Verification items for the finished model (mm, model axes). Give positions to 0.01 mm unless a question says otherwise; leave off trailing zeros. Write each loop counter-clockwise with the first axis right and the second up, starting at its lowest first coordinate (ties: lowest second). Pieces come first, ordered by that corner, then holes. Notation, with made-up numbers: (78.25, -37) - (105.25, -37) arc R15 cw to (105.25, -19) - close; hole circle Ø4 at (-28, 38). An arc over 180 degrees is marked (long way). Put each result on its own line as item: value.
Autodesk Inventor part; units mm, degrees
ref_plane "YZ Plane" through (0, 0, 0) normal (1, 0, 0) x (0, 1, 0)
ref_plane "XZ Plane" through (0, 0, 0) normal (0, 1, 0) x (-1, 0, 0)
ref_plane "XY Plane" through (0, 0, 0) normal (0, 0, 1) x (1, 0, 0)
sketch "Sketch1" plane through (0, 0, 0) normal (0, 1, 0) x (-1, 0, 0)
  circle A0 centre (0, 0) radius 25
  circle A1 centre (0, 0) radius 3
  circle A2 centre (0, 18.36) radius 1
  circle A3 centre (-12.9825, 12.9825) radius 1
  circle A4 centre (-18.36, 0) radius 1
  circle A5 centre (-12.9825, -12.9825) radius 1
  circle A6 centre (0, -18.36) radius 1
  circle A7 centre (12.9825, -12.9825) radius 1
  circle A8 centre (18.36, 0) radius 1
  circle A9 centre (12.9825, 12.9825) radius 1
  dimension "d0" = 50
  dimension "d1" = 6
  dimension "d2" = 2
  dimension "d3" = 18.36
  dimension "d6" = 360
extrude "Extrusion1" add sketch "Sketch1" along normal blind 1.6
properties part number "CUT_FR4_Bottom_Cone_PCB"
Q1. Release check for a two-part mould opening along X. For faces 1 (the face through (0, 1.6, -5)), 2 (the face through (0.13, 0.79, 17.37)), 3 (the face through (-13.52, 0.79, 12.14)), 4 (the face through (-23.846, 0.789, -7.509)) record: released by +X, released by -X, zero draft, split by the parting line, or undercut.
Answers follow:
face 1: zero draft
face 2: undercut
face 3: undercut
face 4: split by the parting line
Q2. Scan lines: line 1 along Z through (x, y) = (0, 0.95); line 2 along X through (y, z) = (0.55, 13); line 3 along X through (y, z) = (0.35, -17.5). Record each from-to range of solid material in increasing order.
Answers follow:
line 1: z = -25 to -19.36, -17.36 to -3, 3 to 17.36, 19.36 to 25
line 2: x = -21.35 to -13.98, -11.98 to 11.98, 13.98 to 21.35
line 3: x = -17.85 to -0.51, 0.51 to 17.85
Q3. Section check D-D, the plane z = -18.36. Record the cut outline in (x, y), plus the area to 3 significant figures.
Answers follow:
outline: (-16.97, 0) - (-1, 0) - (-1, 1.6) - (-16.97, 1.6) - close; (1, 0) - (16.97, 0) - (16.97, 1.6) - (1, 1.6) - close
area: 51.1 mm2
Q4. Go/stop test with a flat-tipped pin: pin 1 Ø9.5 at (x, z) = (0, 0) entering from -Y. Record where the tip stops, or that it passes through.
Answers follow:
pin 1: stops at y = 0
Q5. Section check C-C, the plane y = 0.95. Give the number of separate pieces and of enclosed holes in the cut face, plus the area to 3 significant figures.
Answers follow:
separate pieces: 1
enclosed holes: 9
area: 1,910 mm2
Q6. Section check B-B, the plane z = 0. Record the cut outline in (x, y).
Answers follow:
outline: (-25, 0) - (-19.36, 0) - (-19.36, 1.6) - (-25, 1.6) - close; (-17.36, 0) - (-3, 0) - (-3, 1.6) - (-17.36, 1.6) - close; (3, 0) - (17.36, 0) - (17.36, 1.6) - (3, 1.6) - close; (19.36, 0) - (25, 0) - (25, 1.6) - (19.36, 1.6) - close
Q7. Section check A-A, the plane x = -18.36. Record the cut outline in (y, z), plus the area to 3 significant figures.
Answers follow:
outline: (0, -16.97) - (1.6, -16.97) - (1.6, -1) - (0, -1) - close; (0, 1) - (1.6, 1) - (1.6, 16.97) - (0, 16.97) - close
area: 51.1 mm2
